Check sheet for the modelled part. Datum: model origin and axes. Units: mm. Round coordinates to 2 decimals unless told otherwise and drop trailing zeros. Write each loop counter-clockwise with the first axis right and the second up, starting at its lowest first coordinate (ties: lowest second). Pieces come first, ordered by that corner, then holes. Notation, with made-up numbers: (41.25, -5) - (63.25, -5) arc R18 ccw to (63.25, 30) - close; hole circle Ø1 at (83, 88.5). An arc over 180 degrees is marked (long way). Answer as a JSON object with one key per item and string values. Group by question number.
Item 1: Thickness scan on line 1 (Y direction, x = 29.75, z = 0); line 2 (X direction, y = -793, z = -24); line 3 (Z direction, x = -28, y = -1085). Record the ranges inside material, lowest first.
Item 2: Sectioned sample at A-A on x = 8. Record the boundary of the cut face in (y, z), plus the area to 3 significant figures.
Item 3: Sectioned sample at B-B on y = -391. Record the boundary of the cut face in (x, z).
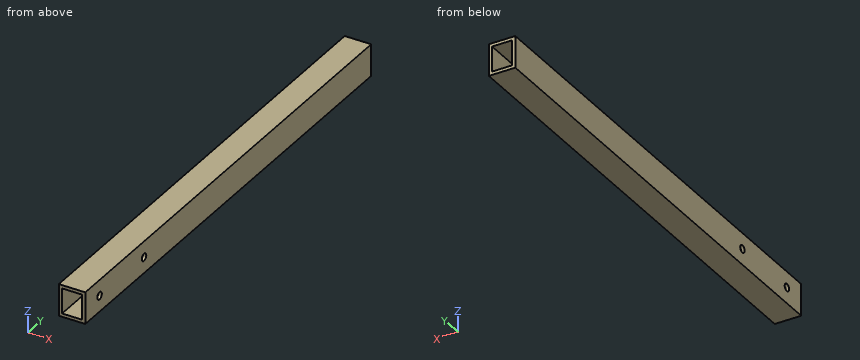
```python
from build123d import *

# Parameters (mm, degrees)
SKETCH1_W           = 63.5
SKETCH1_H           = 76.2
BOSS_EXTRUDE1_DEPTH = 1143
SKETCH2_W           = 47.625
SKETCH2_H           = 60.325
CUT_EXTRUDE1_DEPTH  = 1145.075466261
SKETCH3_R           = 8.89
CUT_EXTRUDE2_DEPTH  = 1146.396376806


with BuildPart() as part:
    # Sketch1 → Boss-Extrude1 (new body)
    with BuildSketch(Plane(origin=(0, 0, 0), x_dir=(1, 0, 0), z_dir=(0, 1, 0))):
        Rectangle(SKETCH1_W, SKETCH1_H)
    extrude(amount=-BOSS_EXTRUDE1_DEPTH)

    # Sketch2 → Cut-Extrude1 (cut, through all)
    with BuildSketch(Plane.XZ.offset(1143)):
        Rectangle(SKETCH2_W, SKETCH2_H)
    extrude(amount=-CUT_EXTRUDE1_DEPTH, mode=Mode.SUBTRACT)

    # Sketch3 → Cut-Extrude2 (cut, through all)
    with BuildSketch(Plane.ZY.offset(31.75)):
        with Locations((0, -908.05)):
            Circle(SKETCH3_R)
        with Locations((0, -1085.85)):
            Circle(SKETCH3_R)
    extrude(amount=-CUT_EXTRUDE2_DEPTH, mode=Mode.SUBTRACT)


solid = part.part
```
Completed:
{
 "1": {"line 1": "-1143 to -1094.74, -1076.96 to -916.94, -899.16 to 0", "line 2": "-31.75 to -23.81, 23.81 to 31.75", "line 3": "-38.1 to -8.85, 8.85 to 38.1"},
 "2": {"outline": "(-1143, -38.1) - (0, -38.1) - (0, -30.16) - (-1143, -30.16) - close; (-1143, 30.16) - (0, 30.16) - (0, 38.1) - (-1143, 38.1) - close", "area": "18,100 mm²"},
 "3": {"outline": "(-31.75, -38.1) - (31.75, -38.1) - (31.75, 38.1) - (-31.75, 38.1) - close; hole (-23.81, -30.16) - (23.81, -30.16) - (23.81, 30.16) - (-23.81, 30.16) - close"}
}
